```python
from build123d import *

# Parameters (mm, degrees)
F1_DEPTH = 12.5
F3_DEPTH = 3.15
F4_R     = 4


with BuildPart() as f1:
    # F0 (on Top) → F1 (new body, symmetric)
    with BuildSketch(Plane.XY):
        Polygon((15, 15), (0, 15), (0, 0), (-15, 0), (-15, -15), (15, -15), align=None)
    extrude(amount=F1_DEPTH, both=True)

    # F2 (on Top) → F3 (cut, symmetric)
    with BuildSketch(Plane.XY):
        Polygon((7.5, 15), (0, 15), (0, 0), (-15, 0), (-15, -7.5), (7.5, -7.5), align=None)
    extrude(amount=F3_DEPTH, both=True, mode=Mode.SUBTRACT)

    # F4
    f4_edges = [f1.edges().sort_by_distance(p)[0] for p in [
        (-15, -15, 0),
        (15, -15, 0),
        (15, 15, 0),
        (15, 0, 12.5),
        (0, -15, 12.5),
        (15, 0, -12.5),
        (0, -15, -12.5),
    ]]
    fillet(f4_edges, radius=F4_R)


solid = f1.part
```
The model under review builds one solid part; all positions refer to its coordinate system, in mm. A direction names the side the tool comes from. Give positions to 0.01 mm unless a question says otherwise; leave off trailing zeros. Write each loop counter-clockwise with the first axis right and the second up, starting at its lowest first coordinate (ties: lowest second). Pieces come first, ordered by that corner, then holes. Notation, with made-up numbers: M 84,-20 L 122,-20 A23 cw 122,19 Z; hole C 73.5,-10 d7. An arc over 180 degrees is marked long. Write each question's results on one line, items separated by ' | '. Start each with the question number.
1. Insertion check: pin 1 Ø4 at (y, z) = (12, -2) entering from -X; pin 2 Ø10.5 at (x, z) = (-10.5, -10) entering from +Y; pin 3 Ø2 at (x, z) = (-8, 0.5) entering from +Y. Each pin has a flat end and moves straight along its axis. Give the tip position at first contact, or say it passes through.
2. For faces 1 (the cylindrical face through (-13.797, -13.859, -0.175)), 2 (the flat face through (-7, 0, -8)), 3 (the flat face through (1, 1, -3.15)), list the 3-axis set-ups (+Z, -Z, +X, -X, +Y, -Y) from which the entire face can be reached by the end or side of a thin tool; tool diameter is ignored.
3. We need section B-B (y = 9). Write out the cut boundary in (x, z).
4. For probe 1 along Z at (x, y) = (0.5, 2); probe 2 along Y at (x, z) = (-6.5, 5.5); probe 3 along X at (y, z) = (-1.5, 1.5), list the stretches that pass through material, from the lowest coordinate up. Write a range as [from, to].
5. We need section D-D (z = -1). Write out the cut boundary in (x, y), and give its area (3 significant figures).
6. We need section A-A (z = -6.5). Write out the cut boundary in (x, y).
7. We need section C-C (x = 5.25). Write out the cut boundary in (y, z), and give its area (3 significant figures).
8. Mouldability with a two-part tool opening along Z and no side actions: class faces 4 (the flat face through (8, 15, 0)), 5 (the flat face through (7.5, 4, 0)), 6 (the cylindrical face through (13.859, 2.182, -11.297)), 7 (the cylindrical face through (-1.818, -13.797, 11.359)) as released by +Z, released by -Z, zero draft, split by the parting line, or undercut.
Results found:
1) pin 1: stops at x = 0 | pin 2: stops at y = 0 | pin 3: stops at y = -7.5
2) face 1: +Z, -Z, -X, -Y | face 2: +Z, -Z, -X, +Y | face 3: -X, +Y
3) outline: M 0,-12.5 L 11,-12.5 A4 ccw 15,-8.5 L 15,8.5 A4 ccw 11,12.5 L 0,12.5 L 0,3.15 L 7.5,3.15 L 7.5,-3.15 L 0,-3.15 Z
4) probe 1: z = [-12.5, -3.15], [3.15, 12.5] | probe 2: y = [-15, 0] | probe 3: x = [7.5, 15]
5) outline: M -15,-11 A4 ccw -11,-15 L 11,-15 A4 ccw 15,-11 L 15,11 A4 ccw 11,15 L 7.5,15 L 7.5,-7.5 L -15,-7.5 Z | area: 383 mm^2
6) outline: M -15,-11 A4 ccw -11,-15 L 11,-15 A4 ccw 15,-11 L 15,11 A4 ccw 11,15 L 0,15 L 0,0 L -15,0 Z
7) outline: M -15,-8.5 A4 ccw -11,-12.5 L 15,-12.5 L 15,-3.15 L -7.5,-3.15 L -7.5,3.15 L 15,3.15 L 15,12.5 L -11,12.5 A4 ccw -15,8.5 Z | area: 601 mm^2
8) face 4: zero draft | face 5: undercut | face 6: released by -Z | face 7: released by +Z
